Verification items for this drawing (mm, ordinates from the low corner). A direction names the side the tool comes from. Give positions to 0.01 mm unless a question says otherwise; leave off trailing zeros. Loops run counter-clockwise (first coordinate to the right, second up) from the corner with the lowest first, then second, coordinate; pieces in that order, holes last. Notation, with made-up numbers: (59.25, 15.25) -> (75.25, 15.25) arc R11 ccw to (75.25, 23.25) -> close; hole circle Ø8 at (-7, 67). An arc over 180 degrees is marked (long way). Answer in a Markdown table with one row per item. Add a question column.
Q1. Section check C-C on y = 44. Enter the section's corners in (x, z) (3 decimals).
Q2. Material ranges on probe 1 along Z at (x, y) = (4.25, 6.5) (3 decimals); probe 2 along Z at (x, y) = (4, 42) (3 decimals); probe 3 along X at (y, z) = (45.5, 11.5) (3 decimals), recorded low to high.
Q3. Section check D-D on z = 7.75. Enter the section's corners in (x, y) (3 decimals).
Q4. Section check A-A on z = 11.5. Enter the section's corners in (x, y) (3 decimals).
Q5. Set-up check for the marked faces 4 and 5: record each of +Z, -Z, +X, -X, +Y, -Y from which the full face is reachable in a straight line by a thin tool's end or side.
Q6. Release check for a two-part mould opening along Z. For the marked faces 1, 2 and 3 record: pulls with the +Z half, pulls with the -Z half, needs draft (parallel to the pull), parting line crosses it, or undercut.
Q7. Section check B-B on x = 2. Enter the section's corners in (y, z) (3 decimals).
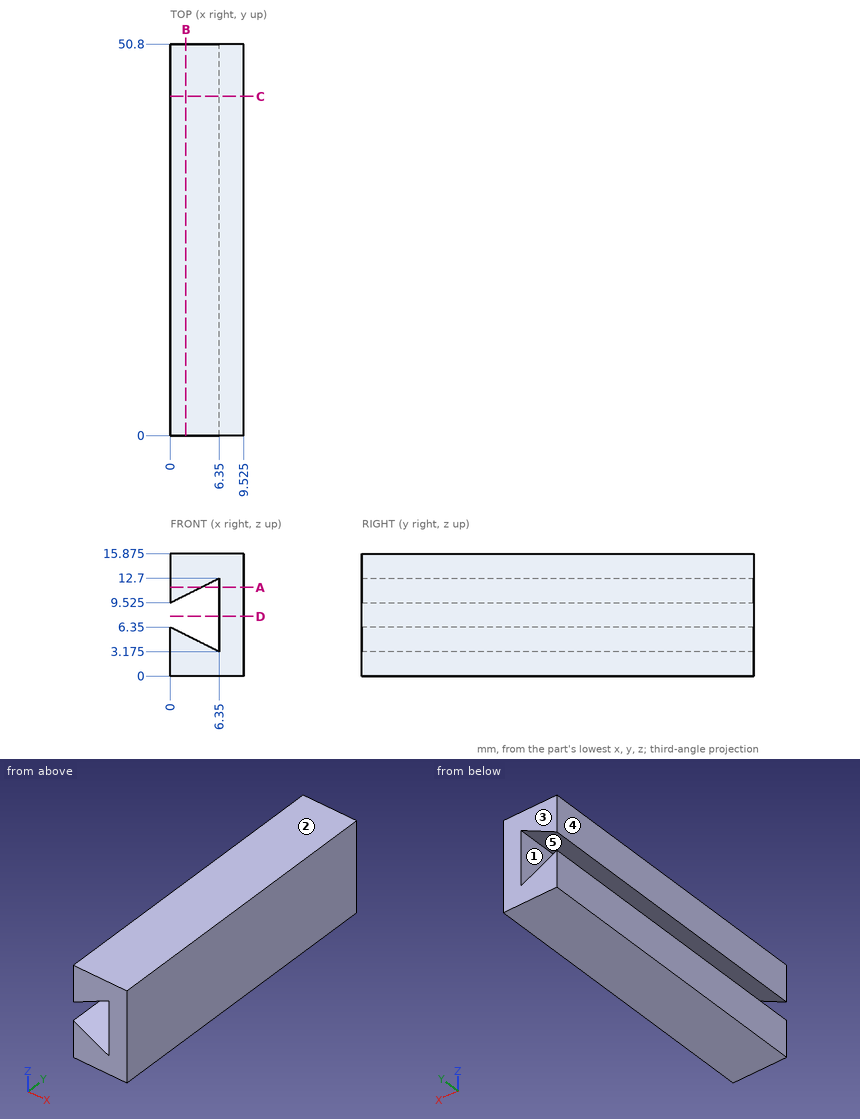
Taken from the geometry:
| question | item | result |
|---|---|---|
| 1 | outline | (0, 0) -> (9.525, 0) -> (9.525, 15.875) -> (0, 15.875) -> (0, 9.525) -> (6.35, 12.7) -> (6.35, 3.175) -> (0, 6.35) -> close |
| 2 | probe 1 | z = 0 to 4.225, 11.65 to 15.875 |
| 2 | probe 2 | z = 0 to 4.35, 11.525 to 15.875 |
| 2 | probe 3 | x = 0 to 3.95, 6.35 to 9.525 |
| 3 | outline | (6.35, 0) -> (9.525, 0) -> (9.525, 50.8) -> (6.35, 50.8) -> close |
| 4 | outline | (0, 0) -> (3.95, 0) -> (3.95, 50.8) -> (0, 50.8) -> close; (6.35, 0) -> (9.525, 0) -> (9.525, 50.8) -> (6.35, 50.8) -> close |
| 5 | face 4 | +Z, -Z, -X, +Y, -Y |
| 5 | face 5 | +Y, -Y |
| 6 | face 1 | undercut |
| 6 | face 2 | pulls with the +Z half |
| 6 | face 3 | needs draft |
| 7 | outline | (0, 0) -> (50.8, 0) -> (50.8, 5.35) -> (0, 5.35) -> close; (0, 10.525) -> (50.8, 10.525) -> (50.8, 15.875) -> (0, 15.875) -> close |
